Verification items for the finished model (mm, model axes). Face numbers are marked on the shaded views. A direction names the side the tool comes from. Round coordinates to 2 decimals unless told otherwise and drop trailing zeros. Write each loop counter-clockwise with the first axis right and the second up, starting at its lowest first coordinate (ties: lowest second). Pieces come first, ordered by that corner, then holes. Notation, with made-up numbers: M 51,16 L 75,16 A7 cw 75,28 Z; hole C 43.5,4.25 d7. An arc over 180 degrees is marked long. Use a Markdown table: item, result. Add a question column.
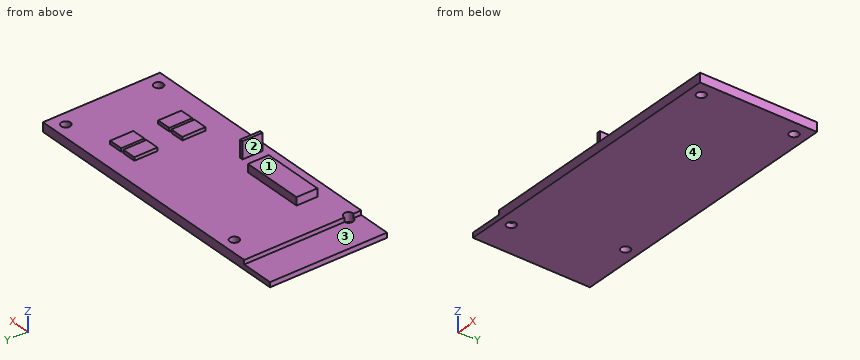
from build123d import *

# Parameters (mm, degrees)
F0_W      = 95
F0_H      = 38.5
F1_DEPTH  = 1.6
F2_W      = 84.2
F2_H      = 38.5
F3_DEPTH  = 1.4
F4_W      = 20.32
F4_H      = 6.858
F5_DEPTH  = 2.6
F6_W      = 4.6
F6_H      = 7.6
F7_DEPTH  = 1.1
F8_W      = 1
F8_H      = 6.6
F9_DEPTH  = 5.6
F10_R     = 1.5
F11_DEPTH = 3


with BuildPart() as f1:
    # F0 (on Top) → F1 (new body)
    with BuildSketch(Plane.XY):
        with Locations((1.023077, 0)):
            Rectangle(F0_W, F0_H)
    extrude(amount=F1_DEPTH)

    # F2 (on face) → F3 (join)
    with BuildSketch(Plane.XY.offset(1.6)):
        with Locations((6.423077, 0)):
            Rectangle(F2_W, F2_H)
    extrude(amount=F3_DEPTH)

    # F4 (on face) → F5 (join)
    with BuildSketch(Plane.XY.offset(3)):
        with Locations((-13.376923, -10.95)):
            Rectangle(F4_W, F4_H)
    extrude(amount=F5_DEPTH)

    # F6 (on face) → F7 (join)
    with BuildSketch(Plane.XY.offset(3)):
        with Locations((27.123077, -7.45)):
            Rectangle(F6_W, F6_H)
        with Locations((21.623077, -7.45)):
            Rectangle(F6_W, F6_H)
        with Locations((21.623077, 8.35)):
            Rectangle(F6_W, F6_H)
        with Locations((27.123077, 8.35)):
            Rectangle(F6_W, F6_H)
    extrude(amount=F7_DEPTH)

    # F8 (on face) → F9 (join)
    with BuildSketch(Plane.XY.offset(3)):
        with Locations((3.043077, -13.55)):
            Rectangle(F8_W, F8_H)
    extrude(amount=F9_DEPTH)

    # F10 (on face) → F11 (cut)
    with BuildSketch(Plane.XY.offset(3)):
        with Locations((-26.476923, 15.25)):
            Circle(F10_R)
        with BuildLine():
            Line((-35.676923, -16.736607), (-35.676923, -13.763393))
            ThreePointArc((-35.676923, -13.763393), (-36.976923, -15.25), (-35.676923, -16.736607))
        make_face()
        with BuildLine():
            ThreePointArc((-35.676923, -16.736607), (-34.489502, -16.379159), (-33.976923, -15.25))
            ThreePointArc((-33.976923, -15.25), (-34.489502, -14.120841), (-35.676923, -13.763393))
            Line((-35.676923, -13.763393), (-35.676923, -16.736607))
        make_face()
        with Locations((44.023077, 15.25)):
            Circle(F10_R)
        with Locations((44.023077, -15.25)):
            Circle(F10_R)
    extrude(amount=-F11_DEPTH, mode=Mode.SUBTRACT)


solid = f1.part
1. Cross-section at B-B on y = -2. Enter the section's corners in (x, z), plus the area to 3 significant figures.
2. Cross-section at C-C on x = 36.5. Enter the section's corners in (y, z).
3. Depth check by flat-ended pin: pin 1 Ø1.1 at (x, z) = (3, 7) entering from +Y; pin 2 Ø2.5 at (x, y) = (-26.48, 15.25) entering from -Z; pin 3 Ø0.9 at (x, z) = (21.5, 3.5) entering from +Y; pin 4 Ø8 at (x, y) = (2.5, 2.5) entering from +Z. Enter the tip coordinate at first touch or a pass-through.
4. Access from +Z, -Z, +X, -X, +Y, -Y to the whole of each face (thin tool, end or side, straight path). Record for the marked faces 3 and 4.
5. Scan lines: line 1 along X through (y, z) = (-11.5, 3.25); line 2 along Z through (x, y) = (-40, -3); line 3 along X through (y, z) = (4, 2.25). Record each from-to range of solid material in increasing order. Write a range as from..to.
6. Release check for a two-part mould opening along X. For the marked faces 1 and 2 record: +X half, -X half, draft (parallel to the pull), parting line (faces both ways), or undercut.
7. Cross-section at A-A on y = 15.25. Enter the section's corners in (x, z), plus the area to 3 significant figures.
Answer:
| question | item | result |
|---|---|---|
| 1 | outline | M -46.48,0 L 48.52,0 L 48.52,3 L -35.68,3 L -35.68,1.6 L -46.48,1.6 Z |
| 1 | area | 270 mm^2 |
| 2 | outline | M -19.25,0 L 19.25,0 L 19.25,3 L -19.25,3 Z |
| 3 | pin 1 | stops at y = -10.25 |
| 3 | pin 2 | passes through |
| 3 | pin 3 | stops at y = 12.15 |
| 3 | pin 4 | stops at z = 3 |
| 4 | face 3 | +Z, -X, +Y, -Y |
| 4 | face 4 | -Z, +X, -X, +Y, -Y |
| 5 | line 1 | x = -23.54..-3.22, 2.54..3.54 |
| 5 | line 2 | z = 0..1.6 |
| 5 | line 3 | x = -35.68..48.52 |
| 6 | face 1 | draft |
| 6 | face 2 | undercut |
| 7 | outline | M -46.48,0 L -27.98,0 L -27.98,3 L -35.68,3 L -35.68,1.6 L -46.48,1.6 Z; M -24.98,0 L 42.52,0 L 42.52,3 L -24.98,3 Z; M 45.52,0 L 48.52,0 L 48.52,3 L 45.52,3 Z |
| 7 | area | 252 mm^2 |
